For this review, take the finished solid that the model builds, in its own axes (mm). A direction names the side the tool comes from. Coordinates: 2 decimals unless noted, no trailing zeros. Write each loop counter-clockwise with the first axis right and the second up, starting at its lowest first coordinate (ties: lowest second). Pieces come first, ordered by that corner, then holes. Notation, with made-up numbers: (14.25, 63.25) - (26.25, 63.25) arc R35 cw to (26.25, 99.25) - close; hole circle Ø9 at (72, 71). An arc over 180 degrees is marked (long way). Use one line per item in the form item = value. Start each with the question number.
1) We need section C-C (x = 29.5). Give the boundary of the cut face in (y, z), plus the area to 3 significant figures.
2) Tool access review of faces 1 (the flat face through (13, 27, -34)), 2 (the flat face through (39, 27, 33)), 3 (the flat face through (13, 27, 33)), 4 (the flat face through (22, 41, 0)), 5 (the flat face through (39, 27, -34)): name each direction out of +Z, -Z, +X, -X, +Y, -Y from which nothing blocks a thin tool from reaching the whole face with its end or side.
3) Mouldability with a two-part tool opening along X and no side actions: class faces 6 (the flat face through (34, 29, -11)), 7 (the flat face through (44, 33, 10)), 8 (the flat face through (12, 23, -22)), 9 (the flat face through (26, 19.5, -28)) as pulls with the +X half, pulls with the -X half, needs draft (parallel to the pull), parting line crosses it, or undercut.
4) For L1, parallel to Y at x = 32, z = -41; L2, parallel to Y at x = 13, z = 0; L3, parallel to Z at x = 34, y = 42.5, list the stretches that pass through material, from the lowest coordinate up. Write a range as from..to.
5) We need section D-D (z = 0). Give the boundary of the cut face in (x, y), plus the area to 3 significant figures.
6) We need section A-A (z = -18). Give the boundary of the cut face in (x, y).
7) We need section B-B (y = 23). Give the boundary of the cut face in (x, z), plus the area to 3 significant figures.
8) Insertion check: P1, Ø18.5, axis at x = 28.5, z = 33, coming from the -Y side; P2, Ø6.5, axis at y = 22.5, z = 34.5, coming from the +X side; P3, Ø10, axis at y = 23.5, z = 11, coming from the +X side; P4, Ø10.5, axis at y = 29.5, z = -34, coming from the -X side. Each pin has a flat end and moves straight along its axis. Give the tip position at first contact, or say it passes through.
```python
from build123d import *

# Parameters (mm, degrees)
SKETCH1_W                = 44
SKETCH1_H                = 46
BOSS_EXTRUDE1_DEPTH      = 22
BOSS_EXTRUDE3_DEPTH      = 23
BOSS_EXTRUDE3_DEPTH_BACK = 67
SKETCH4_W                = 26
SKETCH4_H                = 21
CUT_EXTRUDE1_DEPTH       = 111.236110236
CUT_EXTRUDE1_DEPTH_BACK  = 111.236110236
SKETCH5_W                = 16
SKETCH5_H                = 16
SKETCH6_R                = 12
CUT_EXTRUDE2_DEPTH       = 44
SKETCH7_W                = 28
SKETCH7_H                = 28
CUT_EXTRUDE3_DEPTH       = 5


with BuildPart() as part:
    # Sketch1 → Boss-Extrude1 (new, symmetric)
    with BuildSketch(Plane.XY):
        with Locations((22, 23)):
            Rectangle(SKETCH1_W, SKETCH1_H)
    extrude(amount=BOSS_EXTRUDE1_DEPTH, both=True)

    # Sketch4 → Boss-Extrude3 (add, two sides: drawn at the far end of the back side and taken through both)
    with BuildSketch(Plane.XY.offset(22).offset(-BOSS_EXTRUDE3_DEPTH_BACK)):
        with Locations((26, 27.5)):
            Rectangle(SKETCH4_W, SKETCH4_H)
    extrude(amount=BOSS_EXTRUDE3_DEPTH + BOSS_EXTRUDE3_DEPTH_BACK)

    # Sketch5 → Cut-Extrude1 (cut, two sides: drawn at the far end of the back side and taken through both)
    with BuildSketch(Plane.XY.offset(45).offset(-CUT_EXTRUDE1_DEPTH_BACK)):
        with Locations((26, 27.5)):
            Rectangle(SKETCH5_W, SKETCH5_H)
    extrude(amount=CUT_EXTRUDE1_DEPTH + CUT_EXTRUDE1_DEPTH_BACK, mode=Mode.SUBTRACT)

    # Sketch6 → Cut-Extrude2 (cut)
    with BuildSketch(Plane(origin=(44, 0, 0), x_dir=(0, 0, -1), z_dir=(1, 0, 0))):
        with Locations((0, 23)):
            Circle(SKETCH6_R)
    extrude(amount=-CUT_EXTRUDE2_DEPTH, mode=Mode.SUBTRACT)

    # Sketch7 → Cut-Extrude3 (cut)
    with BuildSketch(Plane(origin=(0, 46, 0), x_dir=(1, 0, 0), z_dir=(0, 1, 0))):
        with Locations((22, 0)):
            Rectangle(SKETCH7_W, SKETCH7_H)
    extrude(amount=-CUT_EXTRUDE3_DEPTH, mode=Mode.SUBTRACT)


solid = part.part
```
Determined:
q1.outline = (0, -22) - (17, -22) - (17, -45) - (19.5, -45) - (19.5, -11.48) arc R12 cw to (19.5, 11.48) - (19.5, 45) - (17, 45) - (17, 22) - (0, 22) - close; (35.5, -45) - (38, -45) - (38, -22) - (46, -22) - (46, -14) - (41, -14) - (41, 14) - (46, 14) - (46, 22) - (38, 22) - (38, 45) - (35.5, 45) - close
q1.area = 1,270 mm²
q2.face_1 = -Z, -X, +Y, -Y
q2.face_2 = +Z, +X, +Y, -Y
q2.face_3 = +Z, -X, +Y, -Y
q2.face_4 = +Y
q2.face_5 = -Z, +X, +Y, -Y
q3.face_6 = undercut
q3.face_7 = pulls with the +X half
q3.face_8 = needs draft
q3.face_9 = undercut
q4.L1 = 17..19.5, 35.5..38
q4.L2 = 0..11, 35..41
q4.L3 = -22..-14, 14..22
q5.outline = (0, 0) - (44, 0) - (44, 11) - (0, 11) - close; (0, 35) - (18, 35) - (18, 35.5) - (34, 35.5) - (34, 35) - (44, 35) - (44, 46) - (36, 46) - (36, 41) - (8, 41) - (8, 46) - (0, 46) - close
q5.area = 820 mm²
q6.outline = (0, 0) - (44, 0) - (44, 46) - (0, 46) - close; hole (18, 19.5) - (34, 19.5) - (34, 35.5) - (18, 35.5) - close
q7.outline = (0, -22) - (13, -22) - (13, -45) - (18, -45) - (18, -12) - (0, -12) - close; (0, 12) - (18, 12) - (18, 45) - (13, 45) - (13, 22) - (0, 22) - close; (34, -45) - (39, -45) - (39, -22) - (44, -22) - (44, -12) - (34, -12) - close; (34, 12) - (44, 12) - (44, 22) - (39, 22) - (39, 45) - (34, 45) - close
q7.area = 1,020 mm²
q8.P1 = 17
q8.P2 = 39
q8.P3 = 44
q8.P4 = 13
